from build123d import *

# Parameters (mm, degrees)
SKETCH1_R           = 11
SKETCH1_R_2         = 4
BOSS_EXTRUDE1_DEPTH = 3.8
SKETCH2_R           = 5
SKETCH2_R_2         = 4
BOSS_EXTRUDE2_DEPTH = 10.8


with BuildPart() as part:
    # Sketch1 → Boss-Extrude1 (new body)
    with BuildSketch(Plane(origin=(0, 0, 0), x_dir=(1, 0, 0), z_dir=(0, 1, 0))):
        with Locations(Location((-3.732448162, -0.493369585, 0), (0, 0, 90))):
            Circle(SKETCH1_R)
        with Locations(Location((-3.732448162, -0.493369585, 0), (0, 0, 90))):
            Circle(SKETCH1_R_2, mode=Mode.SUBTRACT)
    extrude(amount=BOSS_EXTRUDE1_DEPTH)

    # Sketch2 → Boss-Extrude2 (add)
    with BuildSketch(Plane(origin=(0, -4.999999906, 0), x_dir=(-1, 0, 0), z_dir=(0, -1, 0))):
        with Locations(Location((3.732448162, -0.493369585, 0), (0, 0, 90))):
            Circle(SKETCH2_R)
        with Locations(Location((3.732448162, -0.493369585, 0), (0, 0, 90))):
            Circle(SKETCH2_R_2, mode=Mode.SUBTRACT)
    extrude(amount=-BOSS_EXTRUDE2_DEPTH)


solid = part.part
Read the model definition and answer for the solid it produces. Units are mm, in the model's axes. A direction names the side the tool comes from. Coordinates: 2 decimals unless noted, no trailing zeros. Loops run counter-clockwise (first coordinate to the right, second up) from the corner with the lowest first, then second, coordinate; pieces in that order, holes last.
Q1. Consider probe 1 along Y at (x, z) = (-12.75, -4.25); probe 2 along X at (y, z) = (2.5, -1.5); probe 3 along X at (y, z) = (-3.25, 5). Determine where each line is inside the solid, lowest interval first.
Q2. The part is cut by section A-A on x = -5.5. Write down the section's boundary in (y, z).
Q3. The part is cut by section C-C on x = -8. Write down the section's boundary in (y, z), and give its area (3 significant figures).
Q4. Each of these flat-tipped pins is pushed along its axis until it touches: pin 1 Ø6.5 at (x, z) = (-3.73, 0.49) entering from -Y; pin 2 Ø5 at (x, z) = (-1.5, 8.5) entering from -Y; pin 3 Ø2 at (x, y) = (-7.5, 2.5) entering from -Z; pin 4 Ø4 at (y, z) = (4, 8.5) entering from -X. Where does it stop, or does it pass through?
Q5. Which of the six approach directions +Z, -Z, +X, -X, +Y, -Y give full straight-line access (tool end or side, diameter ignored) to faces 1 (the face through (-2.231, -2.535, -4.276)), 2 (the face through (0, 5.8, 3)), 3 (the face through (-1, 3.8, -4))?
Q6. The part is cut by section D-D on y = 1.75. Write down the section's boundary in (x, z), and give its area (3 significant figures).
Q7. The mould has two halves that part along Z. Classify faces 4 (the face through (-2.231, 4.786, -4.276)), 5 (the face through (-1.03, 0.32, 3.44)), 6 (the face through (-1, 0, -4)): +Z half, -Z half, draft (parallel to the pull), parting line (faces both ways), or undercut.
Q8. The part is cut by section B-B on z = 2.75. Write down the section's boundary in (x, y).
Results below:
1. probe 1: y = 0 to 3.8
1. probe 2: x = -14.55 to -7.2, -0.26 to 7.09
1. probe 3: x = -5.9 to -1.57
2. outline: (-5, -4.18) - (0, -4.18) - (0, -10.36) - (3.8, -10.36) - (3.8, -4.18) - (5.8, -4.18) - (5.8, -3.09) - (-5, -3.09) - close; (-5, 4.08) - (5.8, 4.08) - (5.8, 5.17) - (3.8, 5.17) - (3.8, 11.35) - (0, 11.35) - (0, 5.17) - (-5, 5.17) - close
3. outline: (-5, -2.11) - (0, -2.11) - (0, -9.65) - (3.8, -9.65) - (3.8, -2.11) - (5.8, -2.11) - (5.8, 3.1) - (3.8, 3.1) - (3.8, 10.63) - (0, 10.63) - (0, 3.1) - (-5, 3.1) - close
3. area: 114 mm2
4. pin 1: passes through
4. pin 2: stops at y = 0
4. pin 3: stops at z = -10.15
4. pin 4: stops at x = -12.94
5. face 1: -Y
5. face 2: +Z, -Z, +X, -X, +Y
5. face 3: +Y
6. outline: circle Ø22 at (-3.73, 0.49); hole circle Ø8 at (-3.73, 0.49)
6. area: 330 mm2
7. face 4: parting line
7. face 5: undercut
7. face 6: draft
8. outline: (-14.5, 0) - (-8.19, 0) - (-8.19, -5) - (-7.04, -5) - (-7.04, 5.8) - (-8.19, 5.8) - (-8.19, 3.8) - (-14.5, 3.8) - close; (-0.43, -5) - (0.73, -5) - (0.73, 0) - (7.03, 0) - (7.03, 3.8) - (0.73, 3.8) - (0.73, 5.8) - (-0.43, 5.8) - close
